from build123d import *

# Parameters (mm, degrees)
SKETCH_1_W      = 100
SKETCH_1_H      = 67
EXTRUDE_1_DEPTH = 41
SKETCH_2_W      = 100
SKETCH_2_H      = 29
EXTRUDE_2_DEPTH = 20


with BuildPart() as part:
    # 草图1 → 凸台-拉伸1 (new, symmetric)
    with BuildSketch(Plane(origin=(0, 0, 0), x_dir=(0, 0, -1), z_dir=(1, 0, 0))):
        Rectangle(SKETCH_1_W, SKETCH_1_H)
    extrude(amount=EXTRUDE_1_DEPTH, both=True)

    # 草图2 → 凸台-拉伸2 (add)
    with BuildSketch(Plane(origin=(41, 0, 0), x_dir=(0, 0, -1), z_dir=(1, 0, 0))):
        with Locations((0, -19)):
            Rectangle(SKETCH_2_W, SKETCH_2_H)
    extrude(amount=EXTRUDE_2_DEPTH)


solid = part.part
For this review, take the finished solid that the model builds, in its own axes (mm). A direction names the side the tool comes from. Coordinates: 2 decimals unless noted, no trailing zeros. Order: outer loops, then holes, each group sorted by start corner. A loop starts at its lowest first (then second) coordinate and runs counter-clockwise, first axis right, second up. Notation, with made-up numbers: (9.5, 37) - (32.5, 37) arc R21 cw to (32.5, 45) - close; hole circle Ø6 at (69.25, 60). An arc over 180 degrees is marked (long way). Answer as CSV lines item,"result". Start each with the question number.
1) Add section B-B (y = 29.5). State the section outline as (x, z) points.
2) To check wall thickness, follow line 1 along X through (y, z) = (8, -25). State the ranges of the line that lie inside material, in increasing order. Write a range as [from, to].
3) Add section A-A (z = -21). State the section outline as (x, y) points.
4) Machinability: for faces 1 (the flat face through (9, -33.5, 1)), 2 (the flat face through (51, -4.5, 1)), which of the approach directions +Z, -Z, +X, -X, +Y, -Y give a long, thin tool a straight path to every point of the face, cutting with its end or side? Answer none if there is none.
5) Insertion check: P1, Ø16, axis at x = 56, z = 22, coming from the +Y side; P2, Ø19, axis at y = 14.5, z = 12, coming from the +X side. Each pin has a flat end and moves straight along its axis. Give the tip position at first contact, or say it passes through.
Result:
1,outline,"(-41, -50) - (41, -50) - (41, 50) - (-41, 50) - close"
2,line 1,"[-41, 41]"
3,outline,"(-41, -33.5) - (61, -33.5) - (61, -4.5) - (41, -4.5) - (41, 33.5) - (-41, 33.5) - close"
4,face 1,"+Z, -Z, +X, -X, -Y"
4,face 2,"+Z, -Z, +X, +Y"
5,P1,"y = -4.5"
5,P2,"x = 41"
